```python
from build123d import *

# Parameters (mm, degrees)
ESBO_O1_R                = 1.5
RESSALTO_EXTRUS_O1_DEPTH = 3


with BuildPart() as part:
    # Esboço1 → Ressalto-extrusão1 (new body)
    with BuildSketch(Plane.XY):
        Polygon((-24, 100), (24, 100), (24, 50), (94, 50), (94, 37), (100, 37), (100, 27.5), (94, 27.5), (94, -90.5), (100, -90.5), (100, -100), (94, -100), (-94, -100), (-100, -100), (-100, -90.5), (-94, -90.5), (-94, 27.5), (-100, 27.5), (-100, 37), (-94, 37), (-94, 50), (-24, 50), align=None)
        with Locations((97, -95.25)):
            Circle(ESBO_O1_R, mode=Mode.SUBTRACT)
        with Locations((97, 32.25)):
            Circle(ESBO_O1_R, mode=Mode.SUBTRACT)
        with Locations((-97, 32.25)):
            Circle(ESBO_O1_R, mode=Mode.SUBTRACT)
        with Locations((-97, -95.25)):
            Circle(ESBO_O1_R, mode=Mode.SUBTRACT)
    extrude(amount=RESSALTO_EXTRUS_O1_DEPTH)


solid = part.part
```
Model file for the job. Use its own axes, mm. Coordinates: 2 decimals unless noted, no trailing zeros. Write each loop counter-clockwise with the first axis right and the second up, starting at its lowest first coordinate (ties: lowest second). Pieces come first, ordered by that corner, then holes. Notation, with made-up numbers: (10.5, 50) - (36.5, 50) arc R12 cw to (36.5, 61) - close; hole circle Ø9 at (-18, 82). An arc over 180 degrees is marked (long way). Use a Markdown table: item, result. Add a question column.
Item 1: Drill centre lines: line 1 along Y through (x, z) = (97, 2.45); line 2 along X through (y, z) = (-95.25, 1.1); line 3 along X through (y, z) = (4.5, 0.25). Where is each one in solid material? Low to high.
Item 2: Band-saw the part on B-B, the plane y = 20. Write the cut outline in (x, z), and give its area (3 significant figures).
Item 3: Band-saw the part on A-A, the plane z = 2.45. Write the cut outline in (x, y).
Item 4: Drop flat-ended pins along their axis: pin 1 (0.9 mm diameter, centred on x = 97, z = 2, fed in from +Y); pin 2 (5 mm diameter, centred on x = 97, y = 32.25, fed in from +Z); pin 3 (0.9 mm diameter, centred on x = -58, z = 1.5, fed in from +Y). Give the stop position or say it passes through.
Item 5: Band-saw the part on C-C, the plane x = 60. Write the cut outline in (y, z), and give its area (3 significant figures).
A:
| question | item | result |
|---|---|---|
| 1 | line 1 | y = -100 to -96.75, -93.75 to -90.5, 27.5 to 30.75, 33.75 to 37 |
| 1 | line 2 | x = -100 to -98.5, -95.5 to 95.5, 98.5 to 100 |
| 1 | line 3 | x = -94 to 94 |
| 2 | outline | (-94, 0) - (94, 0) - (94, 3) - (-94, 3) - close |
| 2 | area | 564 mm² |
| 3 | outline | (-100, -100) - (100, -100) - (100, -90.5) - (94, -90.5) - (94, 27.5) - (100, 27.5) - (100, 37) - (94, 37) - (94, 50) - (24, 50) - (24, 100) - (-24, 100) - (-24, 50) - (-94, 50) - (-94, 37) - (-100, 37) - (-100, 27.5) - (-94, 27.5) - (-94, -90.5) - (-100, -90.5) - close; hole circle Ø3 at (-97, -95.25); hole circle Ø3 at (-97, 32.25); hole circle Ø3 at (97, -95.25); hole circle Ø3 at (97, 32.25) |
| 4 | pin 1 | stops at y = 37 |
| 4 | pin 2 | stops at z = 3 |
| 4 | pin 3 | stops at y = 50 |
| 5 | outline | (-100, 0) - (50, 0) - (50, 3) - (-100, 3) - close |
| 5 | area | 450 mm² |
